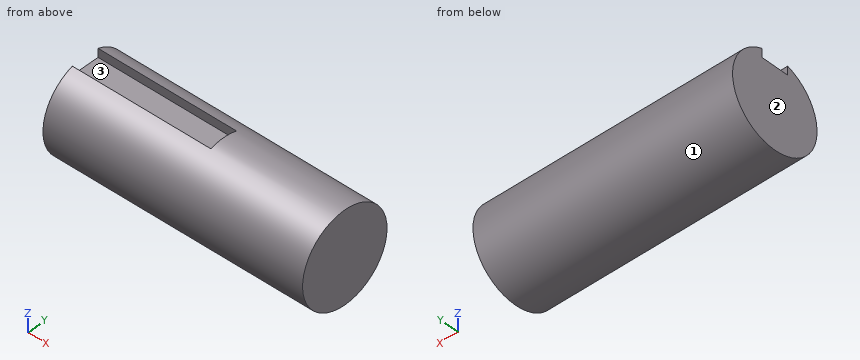
```python
from build123d import *

# Parameters (mm, degrees)
SKETCH1_R           = 52.5
BOSS_EXTRUDE1_DEPTH = 300
CUT_EXTRUDE1_DEPTH  = 160


with BuildPart() as part:
    # Sketch1 → Boss-Extrude1 (new body)
    with BuildSketch(Plane.YZ):
        with Locations(Location((0, 0, 0), (0, 0, 270))):
            Circle(SKETCH1_R)
    extrude(amount=BOSS_EXTRUDE1_DEPTH)

    # Sketch2 → Cut-Extrude1 (cut)
    with BuildSketch(Plane(origin=(0, 0, 0), x_dir=(0, -1, 0), z_dir=(-1, 0, 0))):
        with BuildLine():
            Line((-16, 40.002499938), (16, 40.002499938))
            Line((16, 40.002499938), (16, 50.002499938))
            ThreePointArc((16, 50.002499938), (0, 52.5), (-16, 50.002499938))
            Line((-16, 50.002499938), (-16, 40.002499938))
        make_face()
    extrude(amount=-CUT_EXTRUDE1_DEPTH, mode=Mode.SUBTRACT)


solid = part.part
```
Could you check a few things on this model? Use its own coordinates, in mm. Face numbers are marked on the shaded views. Give positions to 0.01 mm unless a question says otherwise; leave off trailing zeros. Write each loop counter-clockwise with the first axis right and the second up, starting at its lowest first coordinate (ties: lowest second). Pieces come first, ordered by that corner, then holes. Notation, with made-up numbers: (-27, -27.5) -> (-17, -27.5) arc R20 ccw to (-17, -7.5) -> close; hole circle Ø11 at (3.25, 79). An arc over 180 degrees is marked (long way). Write each question's results on one line, items separated by ' | '.
1. I want a section at B-B, the plane z = 44. Write out the boundary of the cut face in (x, y), then the cut area to 3 significant figures.
Check sheet entries:
outline: (0, -28.64) -> (300, -28.64) -> (300, 28.64) -> (0, 28.64) -> (0, 16) -> (160, 16) -> (160, -16) -> (0, -16) -> close | area: 12,100 mm²
2. I need wall thicknesses on L1, parallel to Z at x = 131.5, y = 2.5; L2, parallel to Z at x = 56, y = -27 (3 decimals); L3, parallel to Y at x = 56.5, z = -10. Which ranges of each line are inside material? Lowest first, please.
Check sheet entries:
L1: z = -52.44 to 40 | L2: z = -45.025 to 45.025 | L3: y = -51.54 to 51.54
3. If we mould it in two halves opening along Y, with no side actions, what happens to the marked faces 1, 2 and 3? For each: released by +Y, released by -Y, zero draft, split by the parting line, or undercut.
Check sheet entries:
face 1: split by the parting line | face 2: zero draft | face 3: undercut
4. I want a section at A-A, the plane y = 0. Write out the boundary of the cut face in (x, z).
Check sheet entries:
outline: (0, -52.5) -> (300, -52.5) -> (300, 52.5) -> (160, 52.5) -> (160, 40) -> (0, 40) -> close
5. Will these pins go through, and if not, where does the flat tip stop? pin 1 Ø6 at (y, z) = (-39.5, -28.5) entering from -X; pin 2 Ø2 at (x, y) = (262.5, 9.5) entering from -Z; pin 3 Ø11 at (x, z) = (93, 46) entering from -Y; pin 4 Ø3.5 at (y, z) = (4, 45) entering from -X.
Check sheet entries:
pin 1: stops at x = 0 | pin 2: stops at z = -51.81 | pin 3: stops at y = -33.41 | pin 4: stops at x = 160
6. I want a section at D-D, the plane x = 61. Write out the boundary of the cut face in (y, z), then the cut area to 3 significant figures.
Check sheet entries:
outline: (-16, 40) -> (-16, 50) arc R52.5 ccw (long way) to (16, 50) -> (16, 40) -> close | area: 8,290 mm²
7. I want a section at C-C, the plane x = 236. Write out the boundary of the cut face in (y, z).
Check sheet entries:
outline: circle Ø105 at (0, 0)
